from build123d import *

# Parameters (mm, degrees)
SKETCH1_W                   = 36
SKETCH1_H                   = 38
BOSS_EXTRUDE2_DEPTH         = 53
SKETCH3_W                   = 30
SKETCH3_H                   = 35
CUT_EXTRUDE1_DEPTH          = 51
SKETCH4_W                   = 3
SKETCH4_H                   = 30
BOSS_EXTRUDE3_DEPTH         = 33
SKETCH5_W                   = 53
SKETCH5_H                   = 8
CUT_EXTRUDE2_DEPTH          = 52
SKETCH6_W                   = 53
SKETCH6_H                   = 7
BOSS_EXTRUDE4_DEPTH         = 3
CUT_EXTRUDE4_DEPTH          = 79.797208072
CUT_EXTRUDE4_DEPTH_BACK     = 79.797208072
SKETCH8_W                   = 11.5
SKETCH8_H                   = 3
M3_TAPPED_HOLE1_D           = 2.5
M3_TAPPED_HOLE1_DEPTH       = 3
M3_TAPPED_HOLE1_CSINK_D     = 3.05
M3_TAPPED_HOLE1_CSINK_ANGLE = 179
LPATTERN1_COUNT             = 2
LPATTERN1_PITCH             = 24
LPATTERN1_COUNT_DIR2        = 2
LPATTERN1_PITCH_DIR2        = 12
M3_TAPPED_HOLE2_D           = 2.5
M3_TAPPED_HOLE2_DEPTH       = 2
M3_TAPPED_HOLE2_CSINK_D     = 3.05
M3_TAPPED_HOLE2_CSINK_ANGLE = 179
LPATTERN2_COUNT             = 2
LPATTERN2_PITCH             = 16
LPATTERN2_COUNT_DIR2        = 2
LPATTERN2_PITCH_DIR2        = 12
M3_TAPPED_HOLE3_D           = 2.5
M3_TAPPED_HOLE3_CSINK_D     = 3.05
M3_TAPPED_HOLE3_CSINK_ANGLE = 179
LPATTERN3_COUNT             = 2
LPATTERN3_PITCH             = 16
M3_TAPPED_HOLE4_D           = 2.5
M3_TAPPED_HOLE4_CSINK_D     = 3.05
M3_TAPPED_HOLE4_CSINK_ANGLE = 179
LPATTERN4_COUNT             = 2
LPATTERN4_PITCH             = 24
LPATTERN4_COUNT_DIR2        = 2
LPATTERN4_PITCH_DIR2        = 12
SKETCH45_R                  = 1.833333333
CUT_EXTRUDE5_DEPTH          = 74.396185187
LPATTERN5_COUNT             = 2
LPATTERN5_PITCH             = 35
LPATTERN5_COUNT_DIR2        = 2
LPATTERN5_PITCH_DIR2        = 43
CUT_EXTRUDE6_DEPTH          = 75.551995278
CUT_EXTRUDE6_DEPTH_BACK     = 75.551995278
SKETCH46_W                  = 11.5
SKETCH46_H                  = 3.2


with BuildPart() as part:
    # Sketch1 → Boss-Extrude2 (new body)
    with BuildSketch(Plane(origin=(0, 0, 0), x_dir=(0, 0, -1), z_dir=(1, 0, 0))):
        with Locations((18, 19)):
            Rectangle(SKETCH1_W, SKETCH1_H)
    extrude(amount=BOSS_EXTRUDE2_DEPTH)

    # Sketch3 → Cut-Extrude1 (cut)
    with BuildSketch(Plane(origin=(53, 0, 0), x_dir=(0, 0, -1), z_dir=(1, 0, 0))):
        with Locations((18, 17.5)):
            Rectangle(SKETCH3_W, SKETCH3_H)
    extrude(amount=-CUT_EXTRUDE1_DEPTH, mode=Mode.SUBTRACT)

    # Sketch4 → Boss-Extrude3 (add)
    with BuildSketch(Plane.XY):
        with Locations((51.5, 15)):
            Rectangle(SKETCH4_W, SKETCH4_H)
    extrude(amount=-BOSS_EXTRUDE3_DEPTH)

    # Sketch5 → Cut-Extrude2 (cut)
    with BuildSketch(Plane.XY):
        with Locations((26.5, 34)):
            Rectangle(SKETCH5_W, SKETCH5_H)
    extrude(amount=-CUT_EXTRUDE2_DEPTH, mode=Mode.SUBTRACT)

    # Sketch6 → Boss-Extrude4 (add)
    with BuildSketch(Plane(origin=(0, 0, 0), x_dir=(-1, 0, 0), z_dir=(0, -1, 0))):
        with Locations((-26.5, -3.5)):
            Rectangle(SKETCH6_W, SKETCH6_H)
        with Locations((-26.5, 39.5)):
            Rectangle(SKETCH6_W, SKETCH6_H)
    extrude(amount=-BOSS_EXTRUDE4_DEPTH)

    # Sketch8 → Cut-Extrude4 (cut, two sides: drawn at the far end of the back side and taken through both)
    with BuildSketch(Plane(origin=(0, 0, -43), x_dir=(-1, 0, 0), z_dir=(0, 0, -1)).offset(-CUT_EXTRUDE4_DEPTH_BACK)):
        with Locations((-23.75, 1.5)):
            Rectangle(SKETCH8_W, SKETCH8_H)
    extrude(amount=CUT_EXTRUDE4_DEPTH + CUT_EXTRUDE4_DEPTH_BACK, mode=Mode.SUBTRACT)

    # M3 Tapped Hole1
    with Locations(Plane.XY):
        with Locations((10, 23)):
            m3_tapped_hole1 = CounterSinkHole(M3_TAPPED_HOLE1_D / 2, M3_TAPPED_HOLE1_CSINK_D / 2, depth=M3_TAPPED_HOLE1_DEPTH, counter_sink_angle=M3_TAPPED_HOLE1_CSINK_ANGLE)

    # LPattern1: M3 Tapped Hole1 2 × 2
    with Locations(*[(i * LPATTERN1_PITCH, -j * LPATTERN1_PITCH_DIR2, 0) for i in range(LPATTERN1_COUNT) for j in range(LPATTERN1_COUNT_DIR2) if (i, j) != (0, 0)]):
        add(m3_tapped_hole1, mode=Mode.SUBTRACT)

    # M3 Tapped Hole2
    with Locations(Plane.ZY):
        with Locations((-26, 23)):
            m3_tapped_hole2 = CounterSinkHole(M3_TAPPED_HOLE2_D / 2, M3_TAPPED_HOLE2_CSINK_D / 2, depth=M3_TAPPED_HOLE2_DEPTH, counter_sink_angle=M3_TAPPED_HOLE2_CSINK_ANGLE)

    # LPattern2: M3 Tapped Hole2 2 × 2
    with Locations(*[(0, -j * LPATTERN2_PITCH_DIR2, i * LPATTERN2_PITCH) for i in range(LPATTERN2_COUNT) for j in range(LPATTERN2_COUNT_DIR2) if (i, j) != (0, 0)]):
        add(m3_tapped_hole2, mode=Mode.SUBTRACT)

    # M3 Tapped Hole3 (through all)
    with Locations(Plane(origin=(53, 0, 0), x_dir=(0, 0, -1), z_dir=(1, 0, 0))):
        with Locations((26, 23)):
            m3_tapped_hole3 = CounterSinkHole(M3_TAPPED_HOLE3_D / 2, M3_TAPPED_HOLE3_CSINK_D / 2, counter_sink_angle=M3_TAPPED_HOLE3_CSINK_ANGLE)

    # LPattern3: M3 Tapped Hole3 ×2
    with Locations(*[(0, 0, i * LPATTERN3_PITCH) for i in range(1, LPATTERN3_COUNT)]):
        add(m3_tapped_hole3, mode=Mode.SUBTRACT)

    # M3 Tapped Hole4 (through all)
    with Locations(Plane(origin=(0, 0, -36), x_dir=(-1, 0, 0), z_dir=(0, 0, -1))):
        with Locations((-10, 23)):
            m3_tapped_hole4 = CounterSinkHole(M3_TAPPED_HOLE4_D / 2, M3_TAPPED_HOLE4_CSINK_D / 2, counter_sink_angle=M3_TAPPED_HOLE4_CSINK_ANGLE)

    # LPattern4: M3 Tapped Hole4 2 × 2
    with Locations(*[(i * LPATTERN4_PITCH, -j * LPATTERN4_PITCH_DIR2, 0) for i in range(LPATTERN4_COUNT) for j in range(LPATTERN4_COUNT_DIR2) if (i, j) != (0, 0)]):
        add(m3_tapped_hole4, mode=Mode.SUBTRACT)

    # Sketch45 → Cut-Extrude5 (cut, symmetric)
    with BuildSketch(Plane(origin=(0, 3, 0), x_dir=(1, 0, 0), z_dir=(0, 1, 0))):
        with Locations(Location((8, 39.5, 0), (0, 0, 270))):
            Circle(SKETCH45_R)
    cut_extrude5 = extrude(amount=CUT_EXTRUDE5_DEPTH, both=True, mode=Mode.SUBTRACT)

    # LPattern5: Cut-Extrude5 2 × 2
    with Locations(*[(i * LPATTERN5_PITCH, 0, j * LPATTERN5_PITCH_DIR2) for i in range(LPATTERN5_COUNT) for j in range(LPATTERN5_COUNT_DIR2) if (i, j) != (0, 0)]):
        add(cut_extrude5, mode=Mode.SUBTRACT)

    # Sketch46 → Cut-Extrude6 (cut, two sides: drawn at the far end of the back side and taken through both)
    with BuildSketch(Plane(origin=(0, 0, -36), x_dir=(-1, 0, 0), z_dir=(0, 0, -1)).offset(-CUT_EXTRUDE6_DEPTH_BACK)):
        with Locations((-23.75, 4.6)):
            Rectangle(SKETCH46_W, SKETCH46_H)
    extrude(amount=CUT_EXTRUDE6_DEPTH + CUT_EXTRUDE6_DEPTH_BACK, mode=Mode.SUBTRACT)


solid = part.part
Work out the finished part from the listing and answer in its coordinate system (mm). A direction names the side the tool comes from. Round coordinates to 2 decimals unless told otherwise and drop trailing zeros. Write each loop counter-clockwise with the first axis right and the second up, starting at its lowest first coordinate (ties: lowest second). Pieces come first, ordered by that corner, then holes.
1) Straight lines are drawn through the part: line 1 (Y direction, x = 10, z = -1.5); line 2 (X direction, y = 1, z = 3.5); line 3 (X direction, y = 11, z = -0.7). For each, find the intervals that lie inside material, in ascending order.
2) Given pin 1 Ø8 at (x, y) = (36.5, 17) entering from +Z; pin 2 Ø3 at (x, y) = (13, 22.5) entering from -Z, each flat-ended and moving along its own axis, determine where each tip first touches the part or whether it passes through.
3) A tool of negligible diameter and unlimited length cuts with its end or side. For faces 1 (the flat face through (11, 3, -40)), 2 (the flat face through (50, 15, -18)), 3 (the flat face through (18, 2, 1)), from which of +Z, -Z, +X, -X, +Y, -Y can it reach the whole face along a straight path? Write none if from no direction.
4) A cutting plane is placed at D-D (x = 43). Give the vertices of the cut face in (y, z), plus the area to 3 significant figures.
5) A cutting plane is placed at A-A (z = -26). Give the vertices of the cut face in (x, y) (3 decimals).
6) A cutting plane is placed at C-C (y = 19). Give the vertices of the cut face in (x, z), plus the area to 3 significant figures.
7) A cutting plane is placed at B-B (x = 17). Give the vertices of the cut face in (y, z), plus the area to 3 significant figures.
8) The mould has two halves that part along X. Classify faces 4 (the cylindrical face through (1.015, 11.845, -9.079)), 5 (the cylindrical face through (9.24, 1.52, -40.85)), 6 (the flat face through (53, 15, -18)): pulls with the +X half, pulls with the -X half, needs draft (parallel to the pull), parting line crosses it, or undercut.
Completed:
1. line 1: y = 0 to 9.75, 12.25 to 21.75, 24.25 to 30
1. line 2: x = 0 to 6.17, 9.83 to 18, 29.5 to 41.17, 44.83 to 53
1. line 3: x = 0 to 8.75, 11.25 to 32.75, 35.25 to 53
2. pin 1: stops at z = 0
2. pin 2: stops at z = -36
3. face 1: -Z, +X, -X, +Y
3. face 2: +Y, -Y
3. face 3: +Z, -Z, -Y
4. outline: (0, -43) - (3, -43) - (3, -41.33) - (0, -41.33) - close; (0, -37.67) - (3, -37.67) - (3, -36) - (30, -36) - (30, -33) - (0, -33) - close; (0, -3) - (30, -3) - (30, 0) - (3, 0) - (3, 1.67) - (0, 1.67) - close; (0, 5.33) - (3, 5.33) - (3, 7) - (0, 7) - close
4. area: 200 mm2
5. outline: (0, 0) - (2, 0) - (2, 9.75) - (0.002, 9.75) - (0, 9.475) - close; (0, 12.525) - (0.002, 12.25) - (2, 12.25) - (2, 21.75) - (0.002, 21.75) - (0, 21.475) - close; (0, 24.525) - (0.002, 24.25) - (2, 24.25) - (2, 30) - (0, 30) - close; (50, 0) - (53, 0) - (53, 21.475) - (52.998, 21.75) - (50, 21.75) - close; (50, 24.25) - (52.998, 24.25) - (53, 24.525) - (53, 30) - (50, 30) - close
6. outline: (0, -36) - (53, -36) - (53, 0) - (0, 0) - close; hole (2, -33) - (50, -33) - (50, -3) - (2, -3) - close
6. area: 468 mm2
7. outline: (0, -43) - (3, -43) - (3, -36) - (30, -36) - (30, -33) - (0, -33) - close; (0, -3) - (30, -3) - (30, 0) - (3, 0) - (3, 7) - (0, 7) - close
7. area: 222 mm2
8. face 4: needs draft
8. face 5: undercut
8. face 6: pulls with the +X half
